Build history of the part. All positions in model axes, mm. A direction names the side the tool comes from. Coordinates: 2 decimals unless noted, no trailing zeros. Write each loop counter-clockwise with the first axis right and the second up, starting at its lowest first coordinate (ties: lowest second). Pieces come first, ordered by that corner, then holes.
from build123d import *

# Parameters (mm, degrees)
SKETCH_W        = 54.3
SKETCH_H        = 38.5
PAD_DEPTH       = 2
SKETCH001_W     = 6.85
SKETCH001_H     = 15
PAD001_DEPTH    = 20
SKETCH002_R     = 1.5
POCKET_DEPTH    = 15
PAD002_DEPTH    = 2
FILLET_R        = 3
SKETCH004_R     = 2.45
PAD003_DEPTH    = 6
FILLET001_R     = 1
SKETCH005_R     = 1.5
POCKET001_DEPTH = 5


with BuildPart() as part:
    # Sketch → Pad (new body)
    with BuildSketch(Plane.XY):
        Rectangle(SKETCH_W, SKETCH_H)
    extrude(amount=PAD_DEPTH)

    # Sketch001 (on Face6 of Pad) → Pad001 (join)
    with BuildSketch(Plane.XY.offset(2)):
        with Locations((23.725, -0.95)):
            Rectangle(SKETCH001_W, SKETCH001_H)
        with Locations((-23.725, -0.95)):
            Rectangle(SKETCH001_W, SKETCH001_H)
    extrude(amount=PAD001_DEPTH)

    # Sketch002 (on Face11 of Pad001) → Pocket (cut)
    with BuildSketch(Plane.XZ.offset(8.45)):
        with Locations((24.15, 17)):
            Circle(SKETCH002_R)
        with Locations((24.15, 7)):
            Circle(SKETCH002_R)
        with Locations((-24.15, 17)):
            Circle(SKETCH002_R)
        with Locations((-24.15, 7)):
            Circle(SKETCH002_R)
    extrude(amount=-POCKET_DEPTH, mode=Mode.SUBTRACT)

    # Sketch003 (on Face6 of Pocket) → Pad002 (join)
    with BuildSketch(Plane.XZ.offset(19.25)):
        with BuildLine():
            Line((-27.15, 0), (27.15, 0))
            Line((27.15, 0), (27.15, 22))
            ThreePointArc((27.15, 22), (24.221068, 29.071068), (17.15, 32))
            Line((17.15, 32), (-27.15, 32))
            Line((-27.15, 32), (-27.15, 0))
        make_face()
    extrude(amount=PAD002_DEPTH)

    # Fillet
    fillet_edges = [part.edges().sort_by_distance(p)[0] for p in [
        (27.15, -0.95, 22),
    ]]
    fillet(fillet_edges, radius=FILLET_R)

    # Sketch004 (on Face21 of Fillet) → Pad003 (join)
    with BuildSketch(Plane.XZ.offset(21.25)):
        with Locations((10.1, 12)):
            Circle(SKETCH004_R)
    extrude(amount=PAD003_DEPTH)

    # Fillet001
    fillet001_edges = [part.edges().sort_by_distance(p)[0] for p in [
        (7.65, -27.25, 12),
    ]]
    fillet(fillet001_edges, radius=FILLET001_R)

    # Sketch005 (on Face3 of Fillet001) → Pocket001 (cut)
    with BuildSketch(Plane.XZ.offset(21.25)):
        with Locations((-21.15, 27.5)):
            Circle(SKETCH005_R)
        with Locations((-8.15, 27.5)):
            Circle(SKETCH005_R)
    extrude(amount=-POCKET001_DEPTH, mode=Mode.SUBTRACT)


solid = part.part
(1) Slice it at A-A, the plane x = -8.15. List the corners of the cut face in (y, z).
(2) Flat gauge pins, fed straight in: P1, Ø2.5, axis at x = -24.15, z = 7, coming from the +Y side; P2, Ø2.5, axis at x = -21.15, z = 27.5, coming from the -Y side; P3, Ø3.5, axis at x = 24.15, z = 7, coming from the -Y side; P4, Ø1.9, axis at x = 23, y = 1.5, coming from the +Z side. Where does each tip first touch, or does it go through?
(3) Slice it at D-D, the plane z = 27.5. List the corners of the cut face in (x, y).
(4) Two-plate mould, pull along Z, no slides. Class faces 5 (the cylindrical face through (9.6, -23.7, 9.6)), 6 (the cylindrical face through (25.58, -1.05, 17.45)), 7 (the flat face through (20.3, -1, 12)): pulls with the +Z half, pulls with the -Z half, needs draft (parallel to the pull), parting line crosses it, or undercut.
(5) 3-axis set-ups, long thin cutter, end or side, ignore diameter. For faces 1 (the flat face through (-24, -8.45, 12)), 2 (the cylindrical face through (25.536, -1.055, 6.425)), 3 (the flat face through (-20.3, -1, 12)), 4 (the flat face through (22, -1, 22)): which of +Z, -Z, +X, -X, +Y, -Y reach the whole face in a straight line?
(6) Slice it at C-C, the plane z = 17. List the corners of the cut face in (x, y), and give its area (3 significant figures).
(7) Probe L1, parallel to Z at x = -24, y = 1; L2, parallel to Y at x = 21, z = 19; L3, parallel to X at y = -0.5, z = 12. List the from-to ranges inside material, lowest first.
(8) Slice it at B-B, the plane y = -1. List the corners of the cut face in (x, z), and give its area (3 significant figures).
Results:
1. outline: (-21.25, 0) - (19.25, 0) - (19.25, 2) - (-19.25, 2) - (-19.25, 26) - (-21.25, 26) - close; (-21.25, 29) - (-19.25, 29) - (-19.25, 32) - (-21.25, 32) - close
2. P1: stops at y = -19.25
2. P2: passes through
2. P3: stops at y = -21.25
2. P4: stops at z = 22
3. outline: (-27.15, -21.25) - (-22.65, -21.25) - (-22.65, -19.25) - (-27.15, -19.25) - close; (-19.65, -21.25) - (-9.65, -21.25) - (-9.65, -19.25) - (-19.65, -19.25) - close; (-6.65, -21.25) - (25.5, -21.25) - (25.5, -19.25) - (-6.65, -19.25) - close
4. face 5: parting line crosses it
4. face 6: undercut
4. face 7: needs draft
5. face 1: +Z, +X, -X
5. face 2: +Y
5. face 3: +Z, +Y
5. face 4: +Z, +X, -X, +Y
6. outline: (-27.15, -21.25) - (27.15, -21.25) - (27.15, -19.25) - (-27.15, -19.25) - close; (-27.15, -8.45) - (-25.65, -8.45) - (-25.65, 6.55) - (-27.15, 6.55) - close; (-22.65, -8.45) - (-20.3, -8.45) - (-20.3, 6.55) - (-22.65, 6.55) - close; (20.3, -8.45) - (22.65, -8.45) - (22.65, 6.55) - (20.3, 6.55) - close; (25.65, -8.45) - (27.15, -8.45) - (27.15, 6.55) - (25.65, 6.55) - close
6. area: 224 mm2
7. L1: z = 0 to 5.51, 8.49 to 15.51, 18.49 to 22
7. L2: y = -21.25 to -19.25, -8.45 to 6.55
7. L3: x = -27.15 to -20.3, 20.3 to 27.15
8. outline: (-27.15, 0) - (27.15, 0) - (27.15, 19) arc R3 ccw to (24.15, 22) - (20.3, 22) - (20.3, 2) - (-20.3, 2) - (-20.3, 22) - (-27.15, 22) - close; hole circle Ø3 at (-24.15, 7); hole circle Ø3 at (-24.15, 17); hole circle Ø3 at (24.15, 7); hole circle Ø3 at (24.15, 17)
8. area: 352 mm2
